Geometry: final body of the model. Coordinates: model frame, mm. Face numbers are marked on the shaded views. Round coordinates to 2 decimals unless told otherwise and drop trailing zeros. Write each loop counter-clockwise with the first axis right and the second up, starting at its lowest first coordinate (ties: lowest second). Pieces come first, ordered by that corner, then holes. Notation, with made-up numbers: (39, -4.5) -> (60, -4.5) arc R28 cw to (60, 27.5) -> close; hole circle Ø3 at (76, 6). An arc over 180 degrees is marked (long way). Use one line per item in the form item = value. Start each with the question number.
1. Cut plane B-B, the plane y = -5.5. Return the cut outline in (x, z), plus the area to 3 significant figures.
2. Pin query (flat end, axial travel): pin 1 Ø3 at (x, z) = (-1, 3.5) entering from -Y (3 decimals); pin 2 Ø2 at (x, z) = (-3, 1.5) entering from +Y; pin 3 Ø1.5 at (x, z) = (-4, 4) entering from +Y. Return the tip coordinate at first contact, or that it passes through.
3. Cut plane D-D, the plane y = -11. Return the cut outline in (x, z).
4. Cut plane C-C, the plane x = -17. Return the cut outline in (y, z).
5. Line query: L1, parallel to Y at x = 0.5, z = 1.75 (3 decimals); L2, parallel to Y at x = -3, z = 3.5 (3 decimals); L3, parallel to X at y = 0.5, z = 0.5. Output: solid intervals per line, ascending.
6. Draft query along X for the marked faces 1, 2, 3 and 4. Return one class per face: pulls with the +X half, pulls with the -X half, needs draft (parallel to the pull), parting line crosses it, or undercut.
7. Cut plane A-A, the plane x = 0. Return the cut outline in (y, z) (3 decimals), plus the area to 3 significant figures.
```python
from build123d import *

# Parameters (mm, degrees)
SKETCH1_R             = 22.225
SKETCH1_R_2           = 19.05
BOSS_EXTRUDE1_DEPTH   = 6.35
BOSS_EXTRUDE1_2_DEPTH = 6.35
BOSS_EXTRUDE2_DEPTH   = 6.35
CIRPATTERN1_COUNT     = 3
FILLET2_R             = 1.5875


with BuildPart() as part:
    # Sketch1 → Boss-Extrude1 (new body)
    with BuildSketch(Plane.XY):
        Circle(SKETCH1_R)
        Circle(SKETCH1_R_2, mode=Mode.SUBTRACT)
    extrude(amount=BOSS_EXTRUDE1_DEPTH)



with BuildPart() as body_2:
    # Sketch1 → Boss-Extrude1 2 (new body)
    with BuildSketch(Plane.XY):
        Polygon((-5.499261314, -9.525), (5.499261314, -9.525), (10.998522628, 0), (5.499261314, 9.525), (-5.499261314, 9.525), (-10.998522628, 0), align=None)
        Polygon((3.666174209, -6.35), (7.332348419, 0), (3.666174209, 6.35), (-3.666174209, 6.35), (-7.332348419, 0), (-3.666174209, -6.35), align=None, mode=Mode.SUBTRACT)
    extrude(amount=BOSS_EXTRUDE1_2_DEPTH)


with BuildPart() as part_1:
    add(part.part)

    add(body_2.part)  # Boss-Extrude2 merges body 2
    # Sketch4 → Boss-Extrude2 (add)
    with BuildSketch(Plane.XY):
        with BuildLine():
            Line((-1.5875, 18.98373893), (-1.5875, 9.525))
            Line((-1.5875, 9.525), (1.5875, 9.525))
            Line((1.5875, 9.525), (1.5875, 18.98373893))
            ThreePointArc((1.5875, 18.98373893), (0, 19.05), (-1.5875, 18.98373893))
        make_face()
    boss_extrude2 = extrude(amount=BOSS_EXTRUDE2_DEPTH)

    # CirPattern1: Boss-Extrude2 ×3 about axis
    cirpattern1_axis = Axis((0, 0, 0), (0, 0, 1))
    for i in range(1, CIRPATTERN1_COUNT):
        add(boss_extrude2.rotate(cirpattern1_axis, i * 360 / CIRPATTERN1_COUNT))

    # Fillet2
    fillet2_edges = [part_1.edges().sort_by_distance(p)[0] for p in [
        (-5.499261314, -9.525, 3.175),
        (-10.998522628, 0, 3.175),
        (-5.499261314, 9.525, 3.175),
        (5.499261314, 9.525, 3.175),
        (10.998522628, 0, 3.175),
        (5.499261314, -9.525, 3.175),
        (1.5875, 18.98373893, 3.175),
        (-1.5875, 18.98373893, 3.175),
        (-1.5875, 9.525, 3.175),
        (1.5875, 9.525, 3.175),
        (-17.234150172, -8.117054136, 3.175),
        (-15.646650172, -10.866684793, 3.175),
        (-7.455141971, -6.137315329, 3.175),
        (-9.042641971, -3.387684671, 3.175),
        (15.646650172, -10.866684793, 3.175),
        (17.234150172, -8.117054136, 3.175),
        (9.042641971, -3.387684671, 3.175),
        (7.455141971, -6.137315329, 3.175),
    ]]
    fillet(fillet2_edges, radius=FILLET2_R)


solid = part_1.part
```
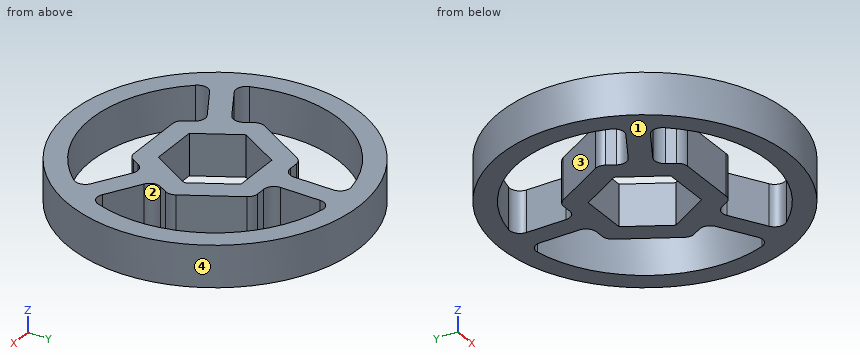
Outcome:
q1.outline = (-21.53, 0) -> (-18.24, 0) -> (-18.24, 6.35) -> (-21.53, 6.35) -> close; (-12.7, 0) -> (-4.16, 0) -> (-4.16, 6.35) -> (-12.7, 6.35) -> close; (4.16, 0) -> (12.7, 0) -> (12.7, 6.35) -> (4.16, 6.35) -> close; (18.24, 0) -> (21.53, 0) -> (21.53, 6.35) -> (18.24, 6.35) -> close
q1.area = 150 mm^2
q2.pin_1 = -22.225
q2.pin_2 = 22.13
q2.pin_3 = 21.99
q3.outline = (-19.31, 0) -> (-14.84, 0) -> (-14.84, 6.35) -> (-19.31, 6.35) -> close; (14.84, 0) -> (19.31, 0) -> (19.31, 6.35) -> (14.84, 6.35) -> close
q4.outline = (-14.32, 0) -> (-7.33, 0) -> (-7.33, 6.35) -> (-14.32, 6.35) -> close; (8.6, 0) -> (14.32, 0) -> (14.32, 6.35) -> (8.6, 6.35) -> close
q5.L1 = -22.219 to -19.043, -9.525 to -6.35, 6.35 to 22.219
q5.L2 = -22.022 to -18.812, -9.525 to -6.35, 6.35 to 9.535, 18.749 to 22.022
q5.L3 = -22.22 to -19.04, -10.67 to -7.04, 7.04 to 10.67, 19.04 to 22.22
q6.face_1 = needs draft
q6.face_2 = undercut
q6.face_3 = undercut
q6.face_4 = parting line crosses it
q7.outline = (-22.225, 0) -> (-19.05, 0) -> (-19.05, 6.35) -> (-22.225, 6.35) -> close; (-9.525, 0) -> (-6.35, 0) -> (-6.35, 6.35) -> (-9.525, 6.35) -> close; (6.35, 0) -> (22.225, 0) -> (22.225, 6.35) -> (6.35, 6.35) -> close
q7.area = 141 mm^2
